from build123d import *

# Parameters (mm, degrees)
BOSS_EXTRUDE2_DEPTH   = 4.7625
F_4_CLEARANCE_HOLE1_D = 3.2639


with BuildPart() as part:
    # Sketch1 → Boss-Extrude2 (new body)
    with BuildSketch(Plane(origin=(0, 0, 0), x_dir=(1, 0, 0), z_dir=(0, 1, 0))):
        with BuildLine():
            Line((-63.5, 6.35), (0, 6.35))
            ThreePointArc((0, 6.35), (6.35, 0), (0, -6.35))
            Line((0, -6.35), (-63.5, -6.35))
            ThreePointArc((-63.5, -6.35), (-69.85, 0), (-63.5, 6.35))
        make_face()
    extrude(amount=BOSS_EXTRUDE2_DEPTH)

    # #4 Clearance Hole1 (through all)
    with Locations(Plane(origin=(0, 4.7625, 0), x_dir=(1, 0, 0), z_dir=(0, 1, 0))):
        with Locations((0, 0)):
            Hole(F_4_CLEARANCE_HOLE1_D / 2)


solid = part.part
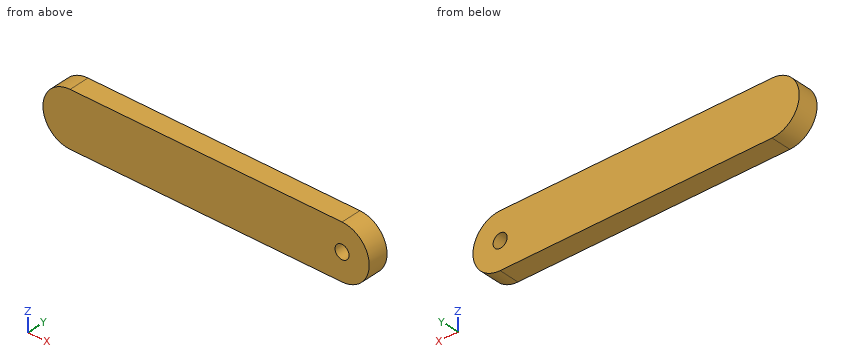
Geometry: final body of the model. Coordinates: model frame, mm. Give positions to 0.01 mm unless a question says otherwise; leave off trailing zeros. Write each loop counter-clockwise with the first axis right and the second up, starting at its lowest first coordinate (ties: lowest second). Pieces come first, ordered by that corner, then holes. Notation, with made-up numbers: M 1,30.5 L 43,30.5 A13 cw 43,39.5 Z; hole C 75.5,-30.5 d9. An arc over 180 degrees is marked long. Answer in a Markdown table with one row per item. Add a question column.
(1) Section B-B on z = 0. Return loops of the section in (x, y), and give its area (3 significant figures).
(2) First-contact query: pin 1 (2 mm diameter, centred on x = 0, z = 0, fed in from +Y). Flat tip, straight axial feed; report the tip coordinate or a pass-through.
(3) Section C-C on z = -5.5. Return loops of the section in (x, y).
(4) Section A-A on y = 2. Return loops of the section in (x, z), and give its area (3 significant figures).
(5) Ray query, line 1 (X direction, y = 0.7, z = -0.25); line 2 (X direction, y = 3.9, z = -2.25); line 3 (X direction, y = 0.8, z = -5.5). Return the intervals inside material, ascending.
Result set:
| question | item | result |
|---|---|---|
| 1 | outline | M -69.85,0 L -1.63,0 L -1.63,4.76 L -69.85,4.76 Z; M 1.63,0 L 6.35,0 L 6.35,4.76 L 1.63,4.76 Z |
| 1 | area | 347 mm^2 |
| 2 | pin 1 | passes through |
| 3 | outline | M -66.67,0 L 3.17,0 L 3.17,4.76 L -66.67,4.76 Z |
| 4 | outline | M -63.5,-6.35 L 0,-6.35 A6.35 ccw 0,6.35 L -63.5,6.35 A6.35 ccw Z; hole C 0,0 d3.26 |
| 4 | area | 925 mm^2 |
| 5 | line 1 | x = -69.85 to -1.61, 1.61 to 6.35 |
| 5 | line 2 | x = -69.44 to 5.94 |
| 5 | line 3 | x = -66.67 to 3.17 |
